Can you work these out from the model? Positions are in its coordinate system, mm. A direction names the side the tool comes from. Give positions to 0.01 mm unless a question says otherwise; leave off trailing zeros. Order: outer loops, then holes, each group sorted by start corner. A loop starts at its lowest first (then second) coordinate and runs counter-clockwise, first axis right, second up. Notation, with made-up numbers: (35, 50) - (90, 50) arc R12 ccw to (90, 73) - close; hole circle Ø6 at (-36, 77). An arc over 180 degrees is marked (long way). Return JSON: item names as keys, results as strings.
```python
from build123d import *

# Parameters (mm, degrees)
F0_R     = 80.01
F1_DEPTH = 101.6
F2_R     = 76.2
F3_DEPTH = 88.9
F4_R     = 5.08
F5_R     = 3.175
F6_DEPTH = 127
F7_R     = 3.175
F8_DEPTH = 127


with BuildPart() as f1:
    # F0 (on Front) → F1 (new body)
    with BuildSketch(Plane.XZ):
        Circle(F0_R)
    extrude(amount=F1_DEPTH)

    # F2 (on face) → F3 (cut)
    with BuildSketch(Plane(origin=(0, 0, 0), x_dir=(-1, 0, 0), z_dir=(0, 1, 0))):
        Circle(F2_R)
    extrude(amount=-F3_DEPTH, mode=Mode.SUBTRACT)

    # F4
    f4_edges = [f1.edges().sort_by_distance(p)[0] for p in [
        (-80.01, -101.6, 0),
    ]]
    fillet(f4_edges, radius=F4_R)

    # F5 (on Top) → F6 (cut, symmetric)
    with BuildSketch(Plane.XY):
        with Locations((0, -50.8)):
            Circle(F5_R)
    extrude(amount=F6_DEPTH, both=True, mode=Mode.SUBTRACT)

    # F7 (on Right) → F8 (cut, symmetric)
    with BuildSketch(Plane.YZ):
        with Locations((-50.8, 0)):
            Circle(F7_R)
    extrude(amount=F8_DEPTH, both=True, mode=Mode.SUBTRACT)


solid = f1.part
```
1. Suppose I cut it at C-C (y = -50.8). List the corners of the cut face in (x, z) for me (3 decimals), plus the area to 3 significant figures.
Checks:
{"outline": "(-79.947, -3.175) arc R80.01 ccw to (-3.175, -79.947) - (-3.175, -76.134) arc R76.2 cw to (-76.134, -3.175) - close; (-79.947, 3.175) - (-76.134, 3.175) arc R76.2 cw to (-3.175, 76.134) - (-3.175, 79.947) arc R80.01 ccw to start; (3.175, -79.947) arc R80.01 ccw to (79.947, -3.175) - (76.134, -3.175) arc R76.2 cw to (3.175, -76.134) - close; (3.175, 76.134) arc R76.2 cw to (76.134, 3.175) - (79.947, 3.175) arc R80.01 ccw to (3.175, 79.947) - close", "area": "1,770 mm^2"}
2. Thinking about a two-plate mould opening in X: for faces 1 (the face through (76.315, -47.584, 24.033)), 2 (the face through (71, 0, -29)), 3 (the face through (1, -88.9, 1)), which applies, +X half, -X half, draft (parallel to the pull), parting line (faces both ways), or undercut?
Checks:
{"face 1": "parting line", "face 2": "draft", "face 3": "undercut"}
3. If I drill on L1, parallel to X at y = -47, z = 0; L2, parallel to Y at x = 26, z = -24, over which ranges is the centre line in solid material (lowest first)? Write a range as [from, to].
Checks:
{"L1": "[-80.01, -76.2], [76.2, 80.01]", "L2": "[-101.6, -88.9]"}
4. Suppose I cut it at B-B (x = 0). List the corners of the cut face in (y, z) for me (3 decimals), plus the area to 3 significant figures.
Checks:
{"outline": "(-101.6, -74.93) arc R5.08 ccw to (-96.52, -80.01) - (-53.975, -80.01) - (-53.975, -76.2) - (-88.9, -76.2) - (-88.9, 76.2) - (-53.975, 76.2) - (-53.975, 80.01) - (-96.52, 80.01) arc R5.08 ccw to (-101.6, 74.93) - close; (-47.625, -80.01) - (0, -80.01) - (0, -76.2) - (-47.625, -76.2) - close; (-47.625, 76.2) - (0, 76.2) - (0, 80.01) - (-47.625, 80.01) - close", "area": "2,650 mm^2"}
5. Suppose I cut it at A-A (z = 0). List the corners of the cut face in (x, y) for me (3 decimals).
Checks:
{"outline": "(-80.01, -96.52) arc R5.08 ccw to (-74.93, -101.6) - (74.93, -101.6) arc R5.08 ccw to (80.01, -96.52) - (80.01, -53.975) - (76.2, -53.975) - (76.2, -88.9) - (-76.2, -88.9) - (-76.2, -53.975) - (-80.01, -53.975) - close; (-80.01, -47.625) - (-76.2, -47.625) - (-76.2, 0) - (-80.01, 0) - close; (76.2, -47.625) - (80.01, -47.625) - (80.01, 0) - (76.2, 0) - close"}
6. For pin 1 Ø8 at (x, y) = (38, -90) entering from +Z; pin 2 Ø1 at (y, z) = (-72, -29.5) entering from -X; pin 3 Ø5.5 at (x, y) = (0, -50.8) entering from -Z; pin 4 Ø2 at (x, y) = (58, -21) entering from -Z, each with a flat end and sliding along its axis, tell me the tip position at first contact or that it passes through.
Checks:
{"pin 1": "z = 72.43", "pin 2": "x = -74.57", "pin 3": "through", "pin 4": "z = -56.15"}
7. On a 3-axis mill with a long thin cutter (end or side, diameter ignored), from which of +Z, -Z, +X, -X, +Y, -Y can I reach the whole of each face in a straight line? I mean faces 4 (the face through (1.707, -48.123, -78.045)), 5 (the face through (60.47, -43.828, -46.367)). Say none if no direction works.
Checks:
{"face 4": "+Z, -Z", "face 5": "+Y"}
